The listing builds one solid part. Answer for the finished solid, in the listing's coordinates (mm). Face numbers are marked on the shaded views. A direction names the side the tool comes from. Give positions to 0.01 mm unless a question says otherwise; leave off trailing zeros. Write each loop counter-clockwise with the first axis right and the second up, starting at its lowest first coordinate (ties: lowest second). Pieces come first, ordered by that corner, then holes.
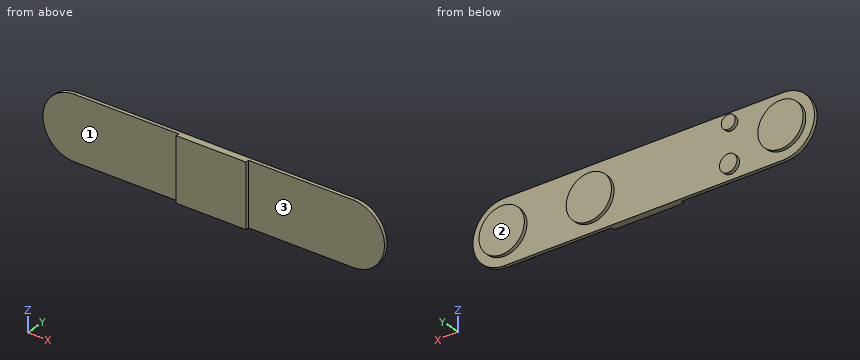
```python
from build123d import *

# Parameters (mm, degrees)
RESSALTO_EXTRUS_O1_DEPTH = 1
ESBO_O2_R                = 2.5
ESBO_O2_R_2              = 2
ESBO_O2_R_3              = 6.5
RESSALTO_EXTRUS_O2_DEPTH = 1
ESBO_O3_W                = 20
ESBO_O3_H                = 18
RESSALTO_EXTRUS_O3_DEPTH = 1


with BuildPart() as part:
    # Esboço1 → Ressalto-extrusão1 (new body)
    with BuildSketch(Plane(origin=(0, 0, 0), x_dir=(1, 0, 0), z_dir=(0, 1, 0))):
        with BuildLine():
            Line((-40, 9), (40, 9))
            ThreePointArc((40, 9), (49, 0), (40, -9))
            Line((40, -9), (-40, -9))
            ThreePointArc((-40, -9), (-49, 0), (-40, 9))
        make_face()
    extrude(amount=RESSALTO_EXTRUS_O1_DEPTH)

    # Esboço2 → Ressalto-extrusão2 (add)
    with BuildSketch(Plane(origin=(0, 1, 0), x_dir=(1, 0, 0), z_dir=(0, 1, 0))):
        with Locations((-25, 5)):
            Circle(ESBO_O2_R)
        with Locations((-25, -6)):
            Circle(ESBO_O2_R_2)
        with Locations((15, 0)):
            Circle(ESBO_O2_R_3)
        with Locations((40, 0)):
            Circle(ESBO_O2_R_3)
        with Locations((-40, 0)):
            Circle(ESBO_O2_R_3)
    extrude(amount=RESSALTO_EXTRUS_O2_DEPTH)

    # Esboço3 → Ressalto-extrusão3 (add)
    with BuildSketch(Plane.XZ):
        Rectangle(ESBO_O3_W, ESBO_O3_H)
    extrude(amount=RESSALTO_EXTRUS_O3_DEPTH)


solid = part.part
```
Item 1: Which of the six approach directions +Z, -Z, +X, -X, +Y, -Y give full straight-line access (tool end or side, diameter ignored) to the marked faces 1, 2 and 3?
Conclusion:
face 1: +Z, -Z, -X, -Y
face 2: +Z, -Z, +X, -X, +Y
face 3: +Z, -Z, +X, -Y
Item 2: A cutting plane is placed at C-C, the plane y = 0.55. Give the vertices of the cut face in (x, z).
Conclusion:
outline: (-40, -9) - (40, -9) arc R9 ccw to (40, 9) - (-40, 9) arc R9 ccw to start
Item 3: Consider probe 1 along X at (y, z) = (1.8, -5.25); probe 2 along X at (y, z) = (1.65, 6); probe 3 along X at (y, z) = (1.5, 3). Determine where each line is inside the solid, lowest interval first.
Conclusion:
probe 1: x = -43.83 to -36.17, -27.49 to -22.51, 11.17 to 18.83, 36.17 to 43.83
probe 2: x = -42.5 to -37.5, -27 to -23, 12.5 to 17.5, 37.5 to 42.5
probe 3: x = -45.77 to -34.23, 9.23 to 20.77, 34.23 to 45.77
Item 4: This flat-tipped pin is pushed along its axis until it touches: P1, Ø1.5, axis at x = 28, z = -0.5, coming from the +Y side. Where does it stop, or does it pass through?
Conclusion:
P1: stops at y = 1
Item 5: A cutting plane is placed at B-B, the plane z = 1.25. Give the vertices of the cut face in (x, y), plus the area to 3 significant figures.
Conclusion:
outline: (-48.91, 0) - (-10, 0) - (-10, -1) - (10, -1) - (10, 0) - (48.91, 0) - (48.91, 1) - (46.38, 1) - (46.38, 2) - (33.62, 2) - (33.62, 1) - (21.38, 1) - (21.38, 2) - (8.62, 2) - (8.62, 1) - (-33.62, 1) - (-33.62, 2) - (-46.38, 2) - (-46.38, 1) - (-48.91, 1) - close
area: 156 mm2
Item 6: A cutting plane is placed at A-A, the plane x = -25. Give the vertices of the cut face in (y, z).
Conclusion:
outline: (0, -9) - (1, -9) - (1, -7.5) - (2, -7.5) - (2, -2.5) - (1, -2.5) - (1, 4) - (2, 4) - (2, 8) - (1, 8) - (1, 9) - (0, 9) - close
Item 7: A cutting plane is placed at D-D, the plane x = 15. Give the vertices of the cut face in (y, z).
Conclusion:
outline: (0, -9) - (1, -9) - (1, -6.5) - (2, -6.5) - (2, 6.5) - (1, 6.5) - (1, 9) - (0, 9) - close
